Autodesk Inventor part; units mm, degrees
ref_plane "YZ Plane" through (0, 0, 0) normal (1, 0, 0) x (0, 1, 0)
ref_plane "XZ Plane" through (0, 0, 0) normal (0, 1, 0) x (-1, 0, 0)
ref_plane "XY Plane" through (0, 0, 0) normal (0, 0, 1) x (1, 0, 0)
sketch "スケッチ1" plane through (0, 0, 0) normal (0, 1, 0) x (-1, 0, 0)
  line L0 (0, 0) -> (0, -43)
  line L1 (0, -43) -> (32, -43)
  line L2 (32, -43) -> (32, 0)
  line L3 (32, 0) -> (0, 0)
  dimension "d0" = 43
  dimension "d1" = 32
extrude "押し出し1" add sketch "スケッチ1" along normal blind 32.5
fillet "フィレット1" radius 2 2 edges at (-32, 16.25, 0) (0, 16.25, 0)
sketch "スケッチ2" plane through (0, 32.5, 0) normal (0, 1, 0) x (1, 0, 0)
  line L0 (0, 43) -> (-32, 43)
  line L1 (-16, 43) -> (-16, 0)
  line L2 (-30, 0) -> (-2, 0)
  line L3 (-16, 21.5) -> (-16, 3)
  line L4 (-16, 3) -> (-2.5, 3)
  line L5 (0, 2) -> (0, 43)
  line L6 (-16, 3) -> (-29.5, 3)
  line L7 (-29.5, 3) -> (-29.5, 30)
  point P0 (0, 0)
  point P1 (-2.5, 30)
  dimension "d5" = 18.5
  dimension "d6" = 13.5
  dimension "d7" = 13.5
  dimension "d8" = 27
hole "穴1" at (-2.5, 32.5, -3) at (-29.5, 32.5, -3) at (-29.5, 32.5, -30) at (-2.5, 32.5, -30) direction (0, -1, 0) diameter 2.6 end through all
sketch "スケッチ3" plane through (0, 32.5, 0) normal (0, 1, 0) x (1, 0, 0)
  line L0 (0, 43) -> (-32, 43)
  line L1 (-16, 43) -> (-16, 0)
  line L2 (-16, 21.5) -> (-16, 31)
  line L3 (-32, 43) -> (-32, 2)
  line L4 (-32, 31) -> (-32, 43)
  line L5 (-32, 43) -> (-26.583, 43)
  line L6 (0, 2) -> (0, 43)
  line L7 (0, 31) -> (0, 43)
  line L8 (0, 43) -> (-5.417, 43)
  arc A0 (-26.583, 43) -> (-32, 31) centre (-16, 31) ccw
  arc A1 (0, 31) -> (-5.417, 43) centre (-16, 31) ccw
  point P0 (0, 0)
  dimension "d16" = 9.5
extrude "押し出し2" cut sketch "スケッチ3" against normal blind 32.5
sketch "スケッチ4" plane through (0, 32.5, 0) normal (0, 1, 0) x (1, 0, 0)
  arc A0 (-26.583, 43) -> (-32, 31) centre (-16, 31) ccw
  circle A1 centre (-16, 31) radius 4
  point P0 (0, 0)
  dimension "d20" = 8
extrude "押し出し3" add sketch "スケッチ4" along normal blind 5
sketch "スケッチ5" plane through (0, 0, 0) normal (0, -1, 0) x (1, 0, 0)
  circle A0 centre (-16, -31) radius 4
  circle A1 centre (-16, -31) radius 4
  point P0 (0, 0)
extrude "押し出し4" add sketch "スケッチ5" along normal blind 5.5
sketch "スケッチ6" plane through (0, 0, 0) normal (0, -1, 0) x (1, 0, 0)
  line L0 (-30, 0) -> (-2, 0)
  line L1 (-16, 0) -> (-1.6, 0)
  line L2 (-1.6, 0) -> (-1.6, 8.5)
  line L3 (-1.6, 0) -> (6.9, 0) construction
  line L4 (-1.6, 8.5) -> (-30.4, 8.5)
  line L5 (-30.4, 8.5) -> (-30.4, -0.1236)
  line L6 (-30.4, -0.1236) -> (-1.6, -0.1236)
  line L7 (-1.6, -0.1236) -> (-1.6, 0)
  point P0 (0, 0)
  dimension "d25" = 14.4
  dimension "d26" = 8.5
  dimension "d27" = 90
  dimension "d28" = 28.8
extrude "押し出し5" add sketch "スケッチ6" against normal blind 11.8
sketch "スケッチ7" plane through (0, 0, 0) normal (0, -1, 0) x (1, 0, 0)
  arc A0 (0, -2) -> (-2, 0) centre (-2, -2) ccw
  arc A1 (-1.6, -0.0404) -> (-2, 0) centre (-2, -2) ccw
  arc A2 (-30.4, -0.0404) -> (-32, -2) centre (-30, -2) ccw
  arc A3 (-30, 0) -> (-30.4, -0.0404) centre (-30, -2) ccw
  line L0 (-1.6, -0.0404) -> (-1.6, 8.5)
  line L1 (-1.6, 8.5) -> (-30.4, 8.5)
  line L2 (-30.4, 8.5) -> (-1.6, 8.5)
  line L3 (-30.4, 8.5) -> (-30.4, -0.0404)
  line L4 (-30, 0) -> (-2, 0)
  arc A4 (-30, 0) -> (-30.4, -0.0404) centre (-30, -2) ccw
  point P0 (0, 0)
extrude "押し出し6" cut sketch "スケッチ7" against normal blind 0.2
thread "ねじ1"
thread "ねじ2"
thread "ねじ3"
thread "ねじ4"
sketch "スケッチ12" plane through (-16, 38, -31) normal (0, 1, 0) x (1, 0, 0)
  circle A0 centre (0, 0) radius 10.5
  point P0 (16, -31)
  dimension "d66" = 21
extrude "押し出し9" add sketch "スケッチ12" against normal blind 5
sketch "スケッチ13" plane through (-16, 38, -31) normal (0, 1, 0) x (1, 0, 0)
  circle A0 centre (0, 0) radius 5
  point P0 (16, -31)
  dimension "d69" = 10
extrude "押し出し10" add sketch "スケッチ13" along normal blind 1
sketch "スケッチ14" plane through (-16, 38, -31) normal (0, 1, 0) x (1, 0, 0)
  circle A0 centre (0, 0) radius 8.5
  circle A1 centre (0, 8.5) radius 1.3
  circle A2 centre (-8.5, 0) radius 1.3
  circle A3 centre (8.5, 0) radius 1.3
  circle A4 centre (0, -8.5) radius 1.3
  point P0 (16, -31)
  dimension "d72" = 17
  dimension "d73" = 2.6
  dimension "d74" = 2.6
  dimension "d75" = 2.6
  dimension "d76" = 2.6
extrude "押し出し11" cut sketch "スケッチ14" against normal blind 5 contours A0 A3 | A0 A3 | A1 A0 | A0 A1 | A4 A0 | A0 A4 | A2 A0 | A0 A2
thread "ねじ9"
thread "ねじ10"
thread "ねじ11"
thread "ねじ12"
sketch "スケッチ15" plane through (0, 0, 0) normal (0, -1, 0) x (1, 0, 0)
  circle A0 centre (-16, -31) radius 4
  circle A1 centre (-16, -31) radius 6
  point P0 (0, 0)
  dimension "d87" = 12
extrude "押し出し12" add sketch "スケッチ15" along normal blind 1.8
sketch "スケッチ16" plane through (-16, -5.5, -31) normal (0, -1, 0) x (1, 0, 0)
  point P0 (16, 31)
  point P1 (0, 0)
hole "穴3" at (-16, -5.5, -31) direction (0, 1, 0) diameter 3 depth 8 tip angle 118
thread "ねじ13"
properties part number "B3M1040" material "アルミニウム 2014-T4"
Here's how the part is built. I have some questions about the finished solid (model axes, mm). A direction names the side the tool comes from. Round coordinates to 2 decimals unless told otherwise and drop trailing zeros. Loops run counter-clockwise (first coordinate to the right, second up) from the corner with the lowest first, then second, coordinate; pieces in that order, holes last.
1. If we section it at A-A on z = -3: Write out the boundary of the cut face in (x, y), plus the area to 3 significant figures.
Answer list:
outline: (-32, 0) - (-30.8, 0) - (-30.8, 32.5) - (-32, 32.5) - close; (-28.2, 0) - (-3.8, 0) - (-3.8, 32.5) - (-28.2, 32.5) - close; (-1.2, 0) - (0, 0) - (0, 32.5) - (-1.2, 32.5) - close
area: 871 mm2
2. For P1, Ø7, axis at y = 6.5, z = 2.5, coming from the -X side; P2, Ø9.5, axis at x = -12, z = -17, coming from the +Y side; P3, Ø4, axis at x = -2.5, z = -30, coming from the -Y side; P4, Ø6, axis at x = -3.5, y = 10.5, coming from the -Z side, each with a flat end and sliding along its axis, tell me the tip position at first contact or that it passes through.
Answer list:
P1: stops at x = -31.73
P2: stops at y = 38
P3: stops at y = 0
P4: stops at z = -43
3. If I drill on line 1 along X through (y, z) = (36.85, -31); line 2 along X through (y, z) = (20, -3); line 3 along Y through (x, z) = (-19, -37), over which ranges is the centre line in solid material (lowest first)?
Answer list:
line 1: x = -26.5 to -25.8, -23.2 to -8.8, -6.2 to -5.5
line 2: x = -32 to -30.8, -28.2 to -3.8, -1.2 to 0
line 3: y = 0 to 32.5, 33 to 38
4. Which directions (+Z, -Z, +X, -X, +Y, -Y) give clear straight access to the entire face, cutting with the end or side of a thin tool? Please do faces 5 (the face through (-11, 33, -31)), 6 (the face through (-30.4, 6, 4)), 7 (the face through (-16.521, -3.624, -34.966)), 8 (the face through (-11, 38, -29)).
Answer list:
face 5: none
face 6: +Z, -X, +Y, -Y
face 7: -Y
face 8: +Y
5. If we section it at D-D on z = -22.5: Write out the boundary of the cut face in (x, y), plus the area to 3 significant figures.
Answer list:
outline: (-32, 0) - (0, 0) - (0, 32.5) - (-32, 32.5) - close; (-22.16, 33) - (-17.3, 33) - (-17.3, 38) - (-22.16, 38) - close; (-14.7, 33) - (-9.84, 33) - (-9.84, 38) - (-14.7, 38) - close
area: 1,090 mm2
6. If we section it at B-B on y = 31: Write out the boundary of the cut face in (x, z).
Answer list:
outline: (-32, -31) arc R16 ccw to (-26.58, -43) - (-5.42, -43) arc R16 ccw to (0, -31) - (0, -2) arc R2 ccw to (-2, 0) - (-30, 0) arc R2 ccw to (-32, -2) - close; hole circle Ø2.6 at (-29.5, -30); hole circle Ø2.6 at (-29.5, -3); hole circle Ø2.6 at (-2.5, -30); hole circle Ø2.6 at (-2.5, -3)
7. We'd pull the mould along X, two halves only. Please class faces 1 (the face through (-16, 32.5, -21)), 2 (the face through (-17.301, -0.887, -25.143)), 3 (the face through (-16.17, 35.53, -40.79)), 4 (the face through (-2.56, 16.02, -31.3)): +X half, -X half, draft (parallel to the pull), parting line (faces both ways), or undercut.
Answer list:
face 1: draft
face 2: parting line
face 3: undercut
face 4: undercut
8. If we section it at C-C on x = -24.5: Write out the boundary of the cut face in (y, z).
Answer list:
outline: (0, -43) - (32.5, -43) - (32.5, 0) - (11.8, 0) - (11.8, 8.5) - (0.2, 8.5) - (0.2, 0) - (0, 0) - close; (33, -37.16) - (38, -37.16) - (38, -32.3) - (33, -32.3) - close; (33, -29.7) - (38, -29.7) - (38, -24.84) - (33, -24.84) - close
